Could you check a few things on this drawing? It's one solid part, dimensions in mm from its lowest x, y, z. A direction names the side the tool comes from. Give positions to 0.01 mm unless a question says otherwise; leave off trailing zeros. Loops run counter-clockwise (first coordinate to the right, second up) from the corner with the lowest first, then second, coordinate; pieces in that order, holes last. Notation, with made-up numbers: (73, -37.75) -> (93, -37.75) arc R15 cw to (93, -33.75) -> close; hole circle Ø1 at (10, -3). An arc over 180 degrees is marked (long way). Use CSV: the item, a comma, the result in double quotes.
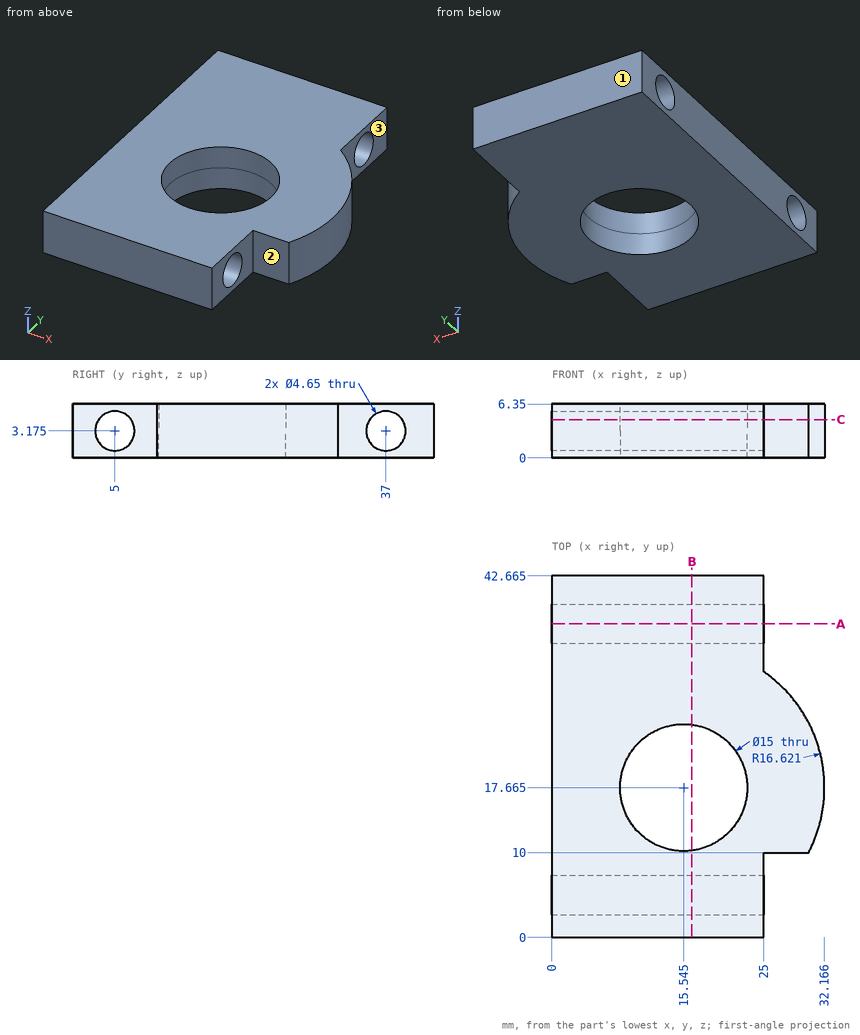
(1) If we section it at C-C, the plane z = 4.5: Write out the boundary of the cut face in (x, y) (1 decimal), then the cut area to 3 significant figures.
Answer sheet:
outline,"(0, 0) -> (25, 0) -> (25, 3.1) -> (0, 3.1) -> close; (0, 6.9) -> (25, 6.9) -> (25, 10) -> (30.3, 10) arc R16.6 ccw to (25, 31.3) -> (25, 35.1) -> (0, 35.1) -> close; (0, 38.9) -> (25, 38.9) -> (25, 42.7) -> (0, 42.7) -> close; hole circle Ø15 at (15.5, 17.7)"
area,"818 mm2"
(2) If we section it at B-B, the plane x = 16.5: Give the number of separate pieces and of enclosed holes in the cut face.
Answer sheet:
separate pieces,"2"
enclosed holes,"2"
(3) If we section it at A-A, the plane y = 37: Write out the boundary of the cut face in (x, z).
Answer sheet:
outline,"(0, 0) -> (25, 0) -> (25, 0.85) -> (0, 0.85) -> close; (0, 5.5) -> (25, 5.5) -> (25, 6.35) -> (0, 6.35) -> close"
(4) Which directions (+Z, -Z, +X, -X, +Y, -Y) give clear straight access to the entire face, cutting with the end or side of a thin tool? Please do the marked faces 1, 2 and 3.
Answer sheet:
face 1,"+Z, -Z, +X, -X, +Y"
face 2,"+Z, -Z, +X, -Y"
face 3,"+Z, -Z, +X, +Y"
(5) Will these pins go through, and if not, where does the flat tip stop? pin 1 Ø3 at (x, y) = (19, 20) entering from -Z; pin 2 Ø1.9 at (y, z) = (3.5, 2.5) entering from +X.
Answer sheet:
pin 1,"passes through"
pin 2,"stops at x = 25"
(6) If I drill on L1, parallel to Y at x = 2, z = 2.5 (1 decimal); L2, parallel to Y at x = 11, z = 3.25 (1 decimal); L3, parallel to Y at x = 2.5, z = 5 (1 decimal), over which ranges is the centre line in solid material (lowest first)? Write a range as from..to.
Answer sheet:
L1,"y = 0..2.8, 7.2..34.8, 39.2..42.7"
L2,"y = 0..2.7, 7.3..11.7, 23.6..34.7, 39.3..42.7"
L3,"y = 0..3.6, 6.4..35.6, 38.4..42.7"
